Autodesk Inventor part; units mm, degrees
ref_plane "Work Plane1" through (39.91, -23.2499, 0) normal (-1, 0, 0) x (0, 0, 1)
ref_plane "YZ Plane" through (0, 0, 0) normal (1, 0, 0) x (0, 1, 0)
ref_plane "XZ Plane" through (0, 0, 0) normal (0, 1, 0) x (-1, 0, 0)
sketch "Sketch1" plane through (0, 0, 0) normal (0, 0, 1) x (1, 0, 0)
  arc A0 (23.7707, 5.756) -> (23.9448, 31.7775) centre (10.4963, 18.8562) ccw
  line L0 (42.91, 38.9085) -> (39.91, 38.8609)
  line L1 (42.91, -0.4) -> (39.91, -0.4)
  line L2 (23.1942, 4.3512) -> (23.1942, 1.6)
  line L3 (39.91, 60.7501) -> (42.91, 60.7501)
  line L4 (42.91, 60.7501) -> (42.91, -23.2499)
  line L5 (42.91, -23.2499) -> (39.91, -23.2499)
  line L6 (39.91, -23.2499) -> (39.91, -0.4)
  line L7 (39.91, 38.8609) -> (39.91, 60.7501)
  line L8 (39.91, -23.2499) -> (39.91, -0.4)
  line L9 (39.91, -0.4) -> (39.91, 60.7501)
  arc A1 (23.1942, 1.6) -> (25.1942, -0.4) centre (25.1942, 1.6) ccw
  arc A2 (23.387, 33.1631) -> (23.9448, 31.7775) centre (25.387, 33.1631) ccw
  arc A3 (23.7707, 5.756) -> (23.1942, 4.3512) centre (25.1942, 4.3512) ccw
  line L10 (39.91, 38.8609) -> (25.3553, 38.63)
  line L11 (39.91, -0.4) -> (25.1942, -0.4)
  line L12 (40.0772, 38.3635) -> (25.3632, 38.13)
  line L13 (23.887, 36.6302) -> (23.887, 33.1631)
  arc A4 (23.887, 33.1631) -> (24.3054, 32.1239) centre (25.387, 33.1631) ccw
  arc A5 (24.1266, 5.4048) -> (24.3054, 32.1239) centre (10.4963, 18.8562) ccw
  arc A6 (24.1266, 5.4048) -> (23.6942, 4.3512) centre (25.1942, 4.3512) ccw
  line L14 (23.6942, 4.3512) -> (23.6942, 1.6)
  arc A7 (23.6942, 1.6) -> (25.1942, 0.1) centre (25.1942, 1.6) ccw
  line L15 (25.1942, 0.1) -> (39.91, 0.1)
  line L16 (39.91, 48.2501) -> (25.887, 48.2501)
  line L17 (23.887, 36.6302) -> (23.887, 46.2501)
  arc A8 (25.887, 48.2501) -> (23.887, 46.2501) centre (25.887, 46.2501) ccw
  point P0 (0, 0)
  point P1 (23.1942, 5.1965)
  point P2 (23.387, 32.334)
  point P3 (36.735, -12.4)
  point P4 (39.91, -12.3999)
  point P5 (39.91, 38.3609)
  dimension "d0" = 3
  dimension "d38" = 2
ref_plane "Work Plane1" through (39.91, -23.2499, 0) normal (-1, 0, 0) x (0, 0, 1)
extrude "Extrusion3" add sketch "Sketch1" along normal blind 32
sketch "Sketch4" plane through (42.91, -23.2499, 0) normal (1, 0, 0) x (0, 0, -1)
  circle A0 centre (-16, 78) radius 3.35
  circle A1 centre (-16, 16.85) radius 3.35
  line L0 (0, 0) -> (0, 84)
  line L1 (-32, 0) -> (-32, 84)
  line L2 (-32, 23.3499) -> (-32, 0)
  line L3 (-32, 10.85) -> (0, 10.85)
  line L4 (0, 23.3499) -> (0, 0)
  line L5 (0, 84) -> (-32, 84)
  line L6 (0, 0) -> (-32, 0)
  line L7 (-32, 0) -> (0, 0)
  line L8 (-16, 84) -> (-16, 10.85) construction
  circle A2 centre (-16, 40.3809) radius 3.3
  point P0 (0, 23.2499)
  dimension "d23" = 6.7
  dimension "d26" = 32
  dimension "d31" = 73.15
  dimension "d33" = 6
  dimension "d34" = 6
  dimension "d39" = 6.6
extrude "Extrusion4" cut sketch "Sketch4" against normal blind 32 contours A0 | A1 | L6 L1 L3 L0 | A2
fillet "Fillet3" radius 2 4 edges at (41.41, 60.7501, 32) (41.41, 60.7501, 0) (41.41, -12.3999, 0) (41.41, -12.3999, 32)
properties part number "Motor Cleat"
Work out the finished part from the listing and answer in its coordinate system (mm). A direction names the side the tool comes from. Give positions to 0.01 mm unless a question says otherwise; leave off trailing zeros. Write each loop counter-clockwise with the first axis right and the second up, starting at its lowest first coordinate (ties: lowest second). Pieces come first, ordered by that corner, then holes. Notation, with made-up numbers: (77, 60.25) - (92, 60.25) arc R18 cw to (92, 82.25) - close; hole circle Ø8 at (-38.5, -12). An arc over 180 degrees is marked (long way). Use one line per item in the form item = value.
1. Each of these flat-tipped pins is pushed along its axis until it touches: pin 1 Ø13.5 at (y, z) = (-8.5, 11.5) entering from -X; pin 2 Ø1.5 at (x, z) = (39, 9) entering from -Y; pin 3 Ø5 at (y, z) = (29, 15.5) entering from -X. Where does it stop, or does it pass through?
Filled in:
pin_1 = 39.91
pin_2 = 0.1
pin_3 = 24.88
2. A cutting plane is placed at C-C (x = 41.75). Write down the section's boundary in (y, z), and give its area (3 significant figures).
Filled in:
outline = (-12.4, 2) arc R2 ccw to (-10.4, 0) - (58.75, 0) arc R2 ccw to (60.75, 2) - (60.75, 30) arc R2 ccw to (58.75, 32) - (-10.4, 32) arc R2 ccw to (-12.4, 30) - close; hole circle Ø6.7 at (-6.4, 16); hole circle Ø6.6 at (17.13, 16); hole circle Ø6.7 at (54.75, 16)
area = 2,230 mm^2
3. A cutting plane is placed at D-D (z = 25.5). Write down the section's boundary in (x, y).
Filled in:
outline = (23.69, 1.6) arc R1.5 ccw to (25.19, 0.1) - (39.91, 0.1) - (39.91, -12.4) - (42.91, -12.4) - (42.91, 60.75) - (39.91, 60.75) - (39.91, 48.25) - (25.89, 48.25) arc R2 ccw to (23.89, 46.25) - (23.89, 33.16) arc R1.5 ccw to (24.31, 32.12) arc R19.15 cw to (24.13, 5.4) arc R1.5 ccw to (23.69, 4.35) - close
4. Determine the mould class of faces 1 (the face through (35, 25, 32)), 2 (the face through (23.694, 3, 16)), 3 (the face through (41.43, 60.15, 0.57)), 4 (the face through (41.43, 51.78, 14.45)) for opening direction Z: released by +Z, released by -Z, zero draft, split by the parting line, or undercut.
Filled in:
face_1 = released by +Z
face_2 = zero draft
face_3 = released by -Z
face_4 = undercut
5. Consider L1, parallel to Y at x = 41.9, z = 16; L2, parallel to Y at x = 38.75, z = 16; L3, parallel to Y at x = 41.5, z = 17. Determine where each line is inside the solid, lowest interval first.
Filled in:
L1 = -12.4 to -9.75, -3.05 to 13.83, 20.43 to 51.4, 58.1 to 60.75
L2 = 0.1 to 13.83, 20.43 to 48.25
L3 = -12.4 to -9.6, -3.2 to 13.99, 20.28 to 51.55, 57.95 to 60.75
6. A cutting plane is placed at A-A (z = 18). Write down the section's boundary in (x, y).
Filled in:
outline = (23.69, 1.6) arc R1.5 ccw to (25.19, 0.1) - (39.91, 0.1) - (39.91, -3.71) - (42.91, -3.71) - (42.91, 14.51) - (29.15, 14.51) arc R19.15 cw to (24.13, 5.4) arc R1.5 ccw to (23.69, 4.35) - close; (23.89, 33.16) arc R1.5 ccw to (24.31, 32.12) arc R19.15 cw to (29.63, 19.76) - (42.91, 19.76) - (42.91, 52.06) - (39.91, 52.06) - (39.91, 48.25) - (25.89, 48.25) arc R2 ccw to (23.89, 46.25) - close; (39.91, -12.4) - (42.91, -12.4) - (42.91, -9.09) - (39.91, -9.09) - close; (39.91, 57.44) - (42.91, 57.44) - (42.91, 60.75) - (39.91, 60.75) - close
7. For faces 5 (the face through (33, 48.25, 16)), 6 (the face through (41.43, 60.18, 31.4)), 7 (the face through (32, 0.1, 16)), determine the directions among +Z, -Z, +X, -X, +Y, -Y from which every point of the face is accessible in a straight line to the end or side of a thin tool.
Filled in:
face_5 = +Z, -Z, -X, +Y
face_6 = +Z, +X, -X, +Y
face_7 = +Z, -Z, -X, -Y
8. A cutting plane is placed at B-B (y = 53). Write down the section's boundary in (x, z), and give its area (3 significant figures).
Filled in:
outline = (39.91, 0) - (42.91, 0) - (42.91, 13.14) - (39.91, 13.14) - close; (39.91, 18.86) - (42.91, 18.86) - (42.91, 32) - (39.91, 32) - close
area = 78.9 mm^2
